Autodesk Inventor part; units mm, degrees
ref_plane "Work Plane2" through (0, 0, 20) normal (0, 0, 1) x (1, 0, 0)
ref_plane "Work Plane8" through (0, 0, 0) normal (0.9510565, 0.309017, 0) x (0, 0, 1)
ref_plane "Work Plane9" through (0, 0, 0) normal (1, 0, 0) x (0, 1, 0)
sketch "Sketch1" plane through (0, 0, 0) normal (0, 0, 1) x (1, 0, 0)
  circle A0 centre (0, 0) radius 12
  dimension "d0" = 24
extrude "Extrusion1" add sketch "Sketch1" along normal blind 40
ref_plane "Work Plane2" through (0, 0, 20) normal (0, 0, 1) x (1, 0, 0)
sketch "Sketch2" plane through (0, 0, 0) normal (0, 0, -1) x (-1, 0, 0)
  circle A0 centre (0, 0) radius 12
  circle A1 centre (0, 0) radius 10
  dimension "d3" = 20
surface extrude "Pitch Diameter" sketch "Sketch2" against normal through all shown no curves A1
ref_plane "Work Plane8" through (0, 0, 0) normal (0.9510565, 0.309017, 0) x (0, 0, 1)
ref_plane "Work Plane9" through (0, 0, 0) normal (1, 0, 0) x (0, 1, 0)
spur gear teeth "Spur Gear" teeth 10 pitch diameter 20 tip diameter 24 root diameter 15 face width 40 start plane through (0, 0, 0) normal (0, 0, -1) x (-1, 0, 0)
equation "\"d0\" = da_da"
equation "\"d1\" = da_b"
equation "\"d3\" = da_d"
equation "\"d16\" = da_aw"
equation "\"d43\" = da_aw"
equation "\"d46\" = da_aw"
properties part number "Spur Gear1" material "Steel"
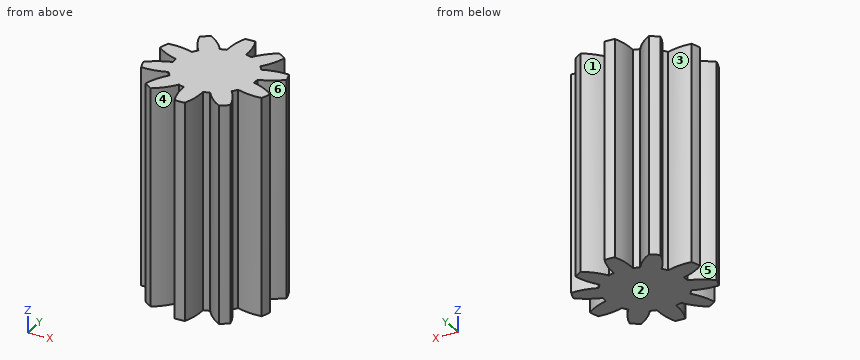
Model file for the job. Use its own axes, mm. Face numbers are marked on the shaded views. A direction names the side the tool comes from. Coordinates: 2 decimals unless noted, no trailing zeros. Loops run counter-clockwise (first coordinate to the right, second up) from the corner with the lowest first, then second, coordinate; pieces in that order, holes last. Notation, with made-up numbers: (35.25, 57) -> (47.25, 57) arc R33 ccw to (47.25, 90) -> close; hole circle Ø6 at (64, 85.5). An arc over 180 degrees is marked (long way). Answer as a JSON object with one key per item and string values.
Q1. Cut at A-A (x = 9.5). List the corners of the cut face in (y, z).
Report:
{"outline": "(-4.6, 0) -> (-1.37, 0) -> (-1.37, 40) -> (-4.6, 40) -> close; (1.37, 0) -> (4.6, 0) -> (4.6, 40) -> (1.37, 40) -> close"}
Q2. Flat gauge pins, fed straight in: P1, Ø6, axis at x = 7.5, z = 19, coming from the +Y side; P2, Ø1.5, axis at x = -9, z = 12.5, coming from the -Y side. Where does each tip first touch, or does it go through?
Report:
{"P1": "stops at y = 10.23", "P2": "stops at y = -4.61"}
Q3. Cut at D-D (y = -6.25). List the corners of the cut face in (x, z), and give its area (3 significant figures).
Report:
{"outline": "(-6.64, 0) -> (6.64, 0) -> (6.64, 40) -> (-6.64, 40) -> close", "area": "531 mm2"}
Q4. Cut at C-C (x = -4.5). List the corners of the cut face in (y, z), and give its area (3 significant figures).
Report:
{"outline": "(-8.87, 0) -> (8.87, 0) -> (8.87, 40) -> (-8.87, 40) -> close", "area": "710 mm2"}
Q5. Probe probe 1 along Y at (x, z) = (6.5, 22); probe 2 along X at (y, z) = (8, 15); probe 3 along Y at (x, z) = (-6.25, 24). List the from-to ranges inside material, lowest first.
Report:
{"probe 1": "y = -10.09 to -6.01, -3.96 to 3.96, 6.01 to 10.09", "probe 2": "x = -7.45 to -3.67, -1.76 to 1.76, 3.67 to 7.45", "probe 3": "y = -10.22 to -5.62, -4.15 to 4.15, 5.62 to 10.22"}
Q6. Cut at B-B (y = 8). List the corners of the cut face in (x, z), and give its area (3 significant figures).
Report:
{"outline": "(-7.45, 0) -> (-3.67, 0) -> (-3.67, 40) -> (-7.45, 40) -> close; (-1.76, 0) -> (1.76, 0) -> (1.76, 40) -> (-1.76, 40) -> close; (3.67, 0) -> (7.45, 0) -> (7.45, 40) -> (3.67, 40) -> close", "area": "443 mm2"}
Q7. Pull direction X, two halves, no side cores. Call the marked faces 4, 5 and 6: released by +X, released by -X, zero draft, split by the parting line, or undercut.
Report:
{"face 4": "undercut", "face 5": "released by -X", "face 6": "released by +X"}
Q8. 3-axis set-ups, long thin cutter, end or side, ignore diameter. For the marked faces 1, 2 and 3: which of +Z, -Z, +X, -X, +Y, -Y reach the whole face in a straight line?
Report:
{"face 1": "+Z, -Z, +Y", "face 2": "-Z, +X, -X, +Y, -Y", "face 3": "+Z, -Z"}
